Read the model definition and answer for the solid it produces. Units are mm, in the model's axes. A direction names the side the tool comes from. Coordinates: 2 decimals unless noted, no trailing zeros. Loops run counter-clockwise (first coordinate to the right, second up) from the corner with the lowest first, then second, coordinate; pieces in that order, holes last.
from build123d import *

# Parameters (mm, degrees)
CUT_EXTRUDE2_DEPTH = 0.85
FILLET1_R          = 1
CHAMFER1_SIZE      = 0.225


with BuildPart() as part:
    # Sketch1 → Revolve1 (revolve)
    with BuildSketch(Plane(origin=(0, 0, 0), x_dir=(0, 0, -1), z_dir=(1, 0, 0))):
        with BuildLine():
            Line((-1.133333333, 2.25), (0, 2.25))
            Line((0, 2.25), (0, 1.25))
            Line((0, 1.25), (4, 1.25))
            Line((4, 1.25), (4, 0))
            Line((4, 0), (-1.7, 0))
            ThreePointArc((-1.7, 0), (-1.556155418, 1.1601305), (-1.133333333, 2.25))
        make_face()
    revolve(axis=Axis((0, 0, 33.735969773), (0, 0, -1)))

    # Sketch2 → Cut-Extrude2 (cut)
    with BuildSketch(Plane(origin=(0, 0, 1.7), x_dir=(-1, 0, 0), z_dir=(0, 0, -1))):
        Polygon((0, 1.3), (0.26, 1.3), (0.26, 0.26), (1.3, 0.26), (1.3, 0), (1.3, -0.26), (0.26, -0.26), (0.26, -1.3), (0, -1.3), (-0.26, -1.3), (-0.26, -0.26), (-1.3, -0.26), (-1.3, 0), (-1.3, 0.26), (-0.26, 0.26), (-0.26, 1.3), align=None)
    extrude(amount=CUT_EXTRUDE2_DEPTH, mode=Mode.SUBTRACT)

    # Fillet1
    fillet1_edges = [part.edges().sort_by_distance(p)[0] for p in [
        (0, -2.25, 1.133333333),
    ]]
    fillet(fillet1_edges, radius=FILLET1_R)

    # Chamfer1
    chamfer1_edges = [part.edges().sort_by_distance(p)[0] for p in [
        (0, -1.25, -4),
    ]]
    chamfer(chamfer1_edges, length=CHAMFER1_SIZE)


solid = part.part
Q1. Straight lines are drawn through the part: probe 1 along X at (y, z) = (1.6, 0.1); probe 2 along X at (y, z) = (-1.25, 1.3); probe 3 along Z at (x, y) = (1.15, -0.6). For each, find the intervals that lie inside material, in ascending order.
Findings below:
probe 1: x = -1.58 to 1.58
probe 2: x = -1.34 to -0.26, 0.26 to 1.34
probe 3: z = 0 to 1.52
Q2. A cutting plane is placed at A-A (z = -0.2). Give the vertices of the cut face in (x, y), then the cut area to 3 significant figures.
Findings below:
outline: circle Ø2.5 at (0, 0)
area: 4.91 mm2
Q3. Which of the six approach directions +Z, -Z, +X, -X, +Y, -Y give full straight-line access (tool end or side, diameter ignored) to faces 1 (the face through (1, -0.26, 1)), 2 (the face through (-1, 1, 0)), 3 (the face through (-0.86, 2.08, 0.24))?
Findings below:
face 1: +Z
face 2: -Z
face 3: +Z, -Z
Q4. Flat-ended cylindrical pins translate along their axes: pin 1 Ø0.7 at (y, z) = (-1, 1) entering from +X; pin 2 Ø0.9 at (y, z) = (-1, 1) entering from -X. Find the tip coordinate at first contact, or state that the pin passes through.
Findings below:
pin 1: stops at x = 2.08
pin 2: stops at x = -2.13
Q5. Determine the mould class of faces 4 (the face through (-1.22, -0.27, -1.91)), 5 (the face through (0, 0, 0.85)), 6 (the face through (0, 0, -4)) for opening direction X: +X half, -X half, draft (parallel to the pull), parting line (faces both ways), or undercut.
Findings below:
face 4: parting line
face 5: undercut
face 6: draft
